The listing builds one solid part. Answer for the finished solid, in the listing's coordinates (mm). A direction names the side the tool comes from. Give positions to 0.01 mm unless a question says otherwise; leave off trailing zeros. Write each loop counter-clockwise with the first axis right and the second up, starting at its lowest first coordinate (ties: lowest second). Pieces come first, ordered by that corner, then holes. Notation, with made-up numbers: (34.25, 35.25) - (50.25, 35.25) arc R29 cw to (50.25, 71.25) - close; hole circle Ø8 at (66.25, 86). An arc over 180 degrees is marked (long way). Return JSON: item names as keys, results as strings.
from build123d import *

# Parameters (mm, degrees)
SKETCH1_W           = 52
SKETCH1_H           = 17
BOSS_EXTRUDE1_DEPTH = 6
BOSS_EXTRUDE2_DEPTH = 6
BOSS_EXTRUDE4_DEPTH = 8
BOSS_EXTRUDE5_DEPTH = 6


with BuildPart() as part:
    # Sketch1 → Boss-Extrude1 (new body)
    with BuildSketch(Plane(origin=(0, 0, 0), x_dir=(1, 0, 0), z_dir=(0, 1, 0))):
        with Locations((-13.173913043, 3.202898551)):
            Rectangle(SKETCH1_W, SKETCH1_H)
    extrude(amount=BOSS_EXTRUDE1_DEPTH)

    # Sketch2 → Boss-Extrude2 (add)
    with BuildSketch(Plane(origin=(0, 6, 0), x_dir=(1, 0, 0), z_dir=(0, 1, 0))):
        Polygon((-39.173913043, 11.702898551), (-26.373913043, 11.702898551), (-26.373913043, 3.365569346), (-30.913828569, 3.365569346), (-30.913828569, -5.297101449), (-39.173913043, -5.297101449), align=None)
    extrude(amount=BOSS_EXTRUDE2_DEPTH)

    # Sketch3 → Boss-Extrude4 (add)
    with BuildSketch(Plane(origin=(0, 6, 0), x_dir=(1, 0, 0), z_dir=(0, 1, 0))):
        Polygon((0.870186747, 11.702898551), (-26.373913043, 11.702898551), (-26.373913043, 3.365569346), (-22.783033953, 3.101787471), (-22.783033953, 8.091138713), (-2.733233594, 8.091138713), (-2.733233594, 3.101787471), (0.870186747, 3.101787471), align=None)
    extrude(amount=BOSS_EXTRUDE4_DEPTH)

    # Sketch4 → Boss-Extrude5 (add)
    with BuildSketch(Plane(origin=(0, 6, 0), x_dir=(1, 0, 0), z_dir=(0, 1, 0))):
        Polygon((0.870186747, 11.702898551), (12.826086957, 11.702898551), (12.826086957, -5.297101449), (4.364373788, -5.297101449), (4.364373788, 3.202898551), (0.870186747, 3.101787471), align=None)
    extrude(amount=BOSS_EXTRUDE5_DEPTH)


solid = part.part
Item 1: A cutting plane is placed at B-B on y = 13.25. Determine the outline of the cut face in (x, z).
Answer below:
{"outline": "(-26.37, -11.7) - (0.87, -11.7) - (0.87, -3.1) - (-2.73, -3.1) - (-2.73, -8.09) - (-22.78, -8.09) - (-22.78, -3.1) - (-26.37, -3.37) - close"}
Item 2: A cutting plane is placed at A-A on z = -7. Determine the outline of the cut face in (x, y).
Answer below:
{"outline": "(-39.17, 0) - (12.83, 0) - (12.83, 12) - (0.87, 12) - (0.87, 14) - (-2.73, 14) - (-2.73, 6) - (-22.78, 6) - (-22.78, 14) - (-26.37, 14) - (-26.37, 12) - (-39.17, 12) - close"}
Item 3: The mould has two halves that part along X. Classify faces 1 (the face through (-39.174, 6, -3)), 2 (the face through (-22.783, 10, -6)), 3 (the face through (-14, 0, -3)): +X half, -X half, draft (parallel to the pull), parting line (faces both ways), or undercut.
Answer below:
{"face 1": "-X half", "face 2": "undercut", "face 3": "draft"}
Item 4: Flat-ended cylindrical pins translate along their axes: P1, Ø1, axis at y = 13, z = -6, coming from the -X side; P2, Ø6.5, axis at x = -14.5, z = -1, coming from the +Y side; P3, Ø4, axis at x = -13.5, y = 11, coming from the +Z side; P4, Ø10, axis at x = -7.5, z = -7, coming from the +Y side. Find the tip coordinate at first contact, or state that the pin passes through.
Answer below:
{"P1": "stops at x = -26.37", "P2": "stops at y = 6", "P3": "stops at z = -8.09", "P4": "stops at y = 14"}
Item 5: Consider L1, parallel to X at y = 10, z = 0.75; L2, parallel to X at y = 7.25, z = -6.5; L3, parallel to Y at x = 5, z = -6. Determine where each line is inside the solid, lowest interval first.
Answer below:
{"L1": "x = -39.17 to -30.91, 4.36 to 12.83", "L2": "x = -39.17 to -22.78, -2.73 to 12.83", "L3": "y = 0 to 12"}
Item 6: For faces 4 (the face through (-34, 12, -3)), 5 (the face through (-24.604, 9.944, -3.236)), 6 (the face through (-13, 5, 5.297)), 7 (the face through (8, 12, -3)), determine the directions among +Z, -Z, +X, -X, +Y, -Y from which every point of the face is accessible in a straight line to the end or side of a thin tool.
Answer below:
{"face 4": "+Z, -Z, -X, +Y", "face 5": "+Z, +Y", "face 6": "+Z, +X, -X, +Y, -Y", "face 7": "+Z, -Z, +X, +Y"}
Item 7: A cutting plane is placed at C-C on x = -19. Determine the outline of the cut face in (y, z), then the cut area to 3 significant figures.
Answer below:
{"outline": "(0, -11.7) - (14, -11.7) - (14, -8.09) - (6, -8.09) - (6, 5.3) - (0, 5.3) - close", "area": "131 mm²"}
Item 8: A cutting plane is placed at D-D on z = -9. Determine the outline of the cut face in (x, y).
Answer below:
{"outline": "(-39.17, 0) - (12.83, 0) - (12.83, 12) - (0.87, 12) - (0.87, 14) - (-26.37, 14) - (-26.37, 12) - (-39.17, 12) - close"}
